Can you work these out from the model? Positions are in its coordinate system, mm. Face numbers are marked on the shaded views. A direction names the side the tool comes from. Coordinates: 2 decimals unless noted, no trailing zeros. Order: outer loops, then holes, each group sorted by start corner. A loop starts at its lowest first (then second) coordinate and runs counter-clockwise, first axis right, second up. Notation, with made-up numbers: (53, 89.5) -> (73, 89.5) arc R15 ccw to (73, 101.5) -> close; hole circle Ø4 at (-9.5, 71.5). An arc over 180 degrees is marked (long way). Answer in a Markdown table with one row per item. Add a question column.
1. Imagine slicing it at B-B on y = 6. Write out the boundary of the cut face in (x, z), plus the area to 3 significant figures.
2. Will these pins go through, and if not, where does the flat tip stop? pin 1 (4 mm diameter, centred on x = -31, z = -14.5, fed in from +Y); pin 2 (2 mm diameter, centred on x = -13, z = -16.5, fed in from +Y); pin 3 (1.1 mm diameter, centred on x = -31, z = 6, fed in from +Y); pin 4 (12 mm diameter, centred on x = 27, y = 19.5, fed in from +Z).
3. On a 3-axis mill with a long thin cutter (end or side, diameter ignored), from which of +Z, -Z, +X, -X, +Y, -Y can I reach the whole of each face in a straight line? I mean the marked faces 1, 2 and 3. Say none if no direction works.
4. Imagine slicing it at A-A on z = -1. Write out the boundary of the cut face in (x, y).
5. If I drill on line 1 along Z through (x, y) = (30.5, -4.25); line 2 along X through (y, z) = (-4, 5.4); line 3 along Z through (x, y) = (-29.5, -5), over which ranges is the centre line in solid material (lowest first)? Write a range as [from, to].
6. Imagine slicing it at D-D on x = 30.5. Write out the boundary of the cut face in (y, z).
7. We'd pull the mould along X, two halves only. Please class the marked faces 4, 5 and 6: pulls with the +X half, pulls with the -X half, needs draft (parallel to the pull), parting line crosses it, or undercut.
8. Imagine slicing it at C-C on x = 0. Write out the boundary of the cut face in (y, z), plus the area to 3 significant figures.
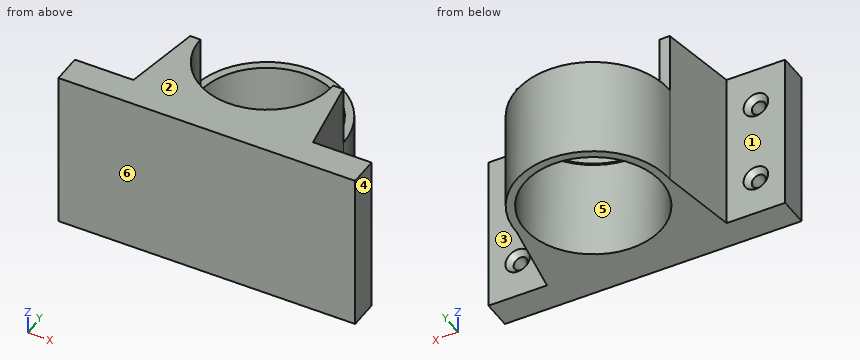
from build123d import *

# Parameters (mm, degrees)
SKETCH1_R                                       = 17.5
BOSS_EXTRUDE9_DEPTH                             = 25.5
BOSS_EXTRUDE10_DEPTH                            = 15.4
BOSS_EXTRUDE10_DEPTH_BACK                       = 25.5
CSK_FOR_M3_FLAT_HEAD_MACHINE_SCREW1_D           = 3.6
CSK_FOR_M3_FLAT_HEAD_MACHINE_SCREW1_CSINK_D     = 6.3
CSK_FOR_M3_FLAT_HEAD_MACHINE_SCREW1_CSINK_ANGLE = 90
CSK_FOR_M3_FLAT_HEAD_MACHINE_SCREW2_D           = 3.6
CSK_FOR_M3_FLAT_HEAD_MACHINE_SCREW2_CSINK_D     = 6.3
CSK_FOR_M3_FLAT_HEAD_MACHINE_SCREW2_CSINK_ANGLE = 90
BOSS_EXTRUDE11_DEPTH                            = 15.4
CUT_EXTRUDE3_REACH                              = 549.129
SKETCH17_R                                      = 1.8
SKETCH18_W                                      = 76
SKETCH18_H                                      = 40.9
BOSS_EXTRUDE12_DEPTH                            = 2.54


with BuildPart() as part:
    # Sketch1 → Boss-Extrude9 (new body)
    with BuildSketch(Plane.XY):
        with BuildLine():
            ThreePointArc((-19.6, 18.153395679), (0, 37.753395679), (19.6, 18.153395679))
            ThreePointArc((19.6, 18.153395679), (0, -1.446604321), (-19.6, 18.153395679))
        make_face()
        with Locations((0, 18.153395679)):
            Circle(SKETCH1_R, mode=Mode.SUBTRACT)
    extrude(amount=-BOSS_EXTRUDE9_DEPTH)

    # Sketch1<15> → Boss-Extrude10 (add, two sides: drawn at the far end of the back side and taken through both)
    with BuildSketch(Plane.XY.offset(-BOSS_EXTRUDE10_DEPTH_BACK)):
        with BuildLine():
            Line((-23, -1.846604321), (-38, -1.846604321))
            Line((-38, -1.846604321), (-38, -6.846604321))
            Line((-38, -6.846604321), (38, -6.846604321))
            Line((38, -6.846604321), (38, -1.846604321))
            Line((38, -1.846604321), (23, -1.846604321))
            Line((23, -1.846604321), (19.6, 18.153395679))
            ThreePointArc((19.6, 18.153395679), (0, -1.446604321), (-19.6, 18.153395679))
            Line((-19.6, 18.153395679), (-23, -1.846604321))
        make_face()
    extrude(amount=BOSS_EXTRUDE10_DEPTH + BOSS_EXTRUDE10_DEPTH_BACK)

    # CSK for M3 Flat Head Machine Screw1 (through all)
    with Locations(Plane(origin=(0, -1.846604321, 0), x_dir=(1, 0, 0), z_dir=(0, 1, 0))):
        with Locations((-30.5, 15.5), (-30.5, -5.4)):
            CounterSinkHole(CSK_FOR_M3_FLAT_HEAD_MACHINE_SCREW1_D / 2, CSK_FOR_M3_FLAT_HEAD_MACHINE_SCREW1_CSINK_D / 2, counter_sink_angle=CSK_FOR_M3_FLAT_HEAD_MACHINE_SCREW1_CSINK_ANGLE)

    # CSK for M3 Flat Head Machine Screw2 (through all)
    with Locations(Plane(origin=(0, -1.846604321, 0), x_dir=(1, 0, 0), z_dir=(0, 1, 0))):
        with Locations((30.5, -5.4), (30.5, 15.5)):
            CounterSinkHole(CSK_FOR_M3_FLAT_HEAD_MACHINE_SCREW2_D / 2, CSK_FOR_M3_FLAT_HEAD_MACHINE_SCREW2_CSINK_D / 2, counter_sink_angle=CSK_FOR_M3_FLAT_HEAD_MACHINE_SCREW2_CSINK_ANGLE)

    # Sketch1<19> → Boss-Extrude11 (add)
    with BuildSketch(Plane.XY):
        with BuildLine():
            ThreePointArc((-19.6, 18.153395679), (0, -1.446604321), (19.6, 18.153395679))
            Line((19.6, 18.153395679), (17, 18.153395679))
            ThreePointArc((17, 18.153395679), (0, 1.153395679), (-17, 18.153395679))
            Line((-17, 18.153395679), (-19.6, 18.153395679))
        make_face()
    extrude(amount=BOSS_EXTRUDE11_DEPTH)

    # Sketch17 → Cut-Extrude3 (cut, up to next)
    with BuildSketch(Plane(origin=(-499.24894984, 9.974554812, -84.308871479), x_dir=(0.050830850863694654, -0.0009181581696580717, 0.9987068546806156), z_dir=(0.0360908865319125, 0.9993480899541042, -0.0009181581696581681)), mode=Mode.PRIVATE) as cut_extrude3_sk1:
        with Locations((92.5, 462.5)):
            Circle(SKETCH17_R)
    cut_extrude3_tool1 = extrude(cut_extrude3_sk1.sketch, amount=-CUT_EXTRUDE3_REACH, mode=Mode.PRIVATE) & part.part
    # Sketch17 → Cut-Extrude3 (cut, up to next)
    with BuildSketch(Plane(origin=(-499.24894984, 9.974554812, -84.308871479), x_dir=(0.050830850863694654, -0.0009181581696580717, 0.9987068546806156), z_dir=(0.0360908865319125, 0.9993480899541042, -0.0009181581696581681)), mode=Mode.PRIVATE) as cut_extrude3_sk2:
        with Locations((113.4, 462.5)):
            Circle(SKETCH17_R)
    cut_extrude3_tool2 = extrude(cut_extrude3_sk2.sketch, amount=-CUT_EXTRUDE3_REACH, mode=Mode.PRIVATE) & part.part
    add(cut_extrude3_tool1.solids().sort_by_distance((-32.946684, -6.80241, -15.437756))[0], mode=Mode.SUBTRACT)
    add(cut_extrude3_tool2.solids().sort_by_distance((-31.884319, -6.821599, 5.435217))[0], mode=Mode.SUBTRACT)

    # Sketch18 → Boss-Extrude12 (add)
    with BuildSketch(Plane.XZ.offset(6.846604321)):
        with Locations((0, -5.05)):
            Rectangle(SKETCH18_W, SKETCH18_H)
    extrude(amount=BOSS_EXTRUDE12_DEPTH)


solid = part.part
Answers follow:
| question | item | result |
|---|---|---|
| 1 | outline | (-21.67, -25.5) -> (-12.59, -25.5) -> (-12.59, 0) -> (-11.89, 0) -> (-11.89, 15.4) -> (-21.67, 15.4) -> close; (11.89, 0) -> (12.59, 0) -> (12.59, -25.5) -> (21.67, -25.5) -> (21.67, 15.4) -> (11.89, 15.4) -> close |
| 1 | area | 764 mm² |
| 2 | pin 1 | stops at y = -1.88 |
| 2 | pin 2 | stops at y = 33.65 |
| 2 | pin 3 | stops at y = -6.85 |
| 2 | pin 4 | passes through |
| 3 | face 1 | +Z, -Z, -X, +Y |
| 3 | face 2 | +Z, +X, -X, +Y, -Y |
| 3 | face 3 | +Z, -Z, +X, +Y |
| 4 | outline | (-38, -9.39) -> (38, -9.39) -> (38, -1.85) -> (23, -1.85) -> (19.6, 18.15) arc R19.6 ccw to (-19.6, 18.15) -> (-23, -1.85) -> (-38, -1.85) -> close; hole circle Ø35 at (0, 18.15) |
| 5 | line 1 | z = [-25.5, -17.3], [-13.7, 3.6], [7.2, 15.4] |
| 5 | line 2 | x = [-38, -32.3], [-28.7, 28.7], [32.3, 38] |
| 5 | line 3 | z = [-25.5, -17], [-14, 3.9], [6.9, 15.4] |
| 6 | outline | (-9.39, -25.5) -> (-1.85, -25.5) -> (-1.85, -18.65) -> (-3.2, -17.3) -> (-6.85, -17.3) -> (-6.85, -13.7) -> (-3.2, -13.7) -> (-1.85, -12.35) -> (-1.85, 2.25) -> (-3.2, 3.6) -> (-6.85, 3.6) -> (-6.85, 7.2) -> (-3.2, 7.2) -> (-1.85, 8.55) -> (-1.85, 15.4) -> (-9.39, 15.4) -> close |
| 7 | face 4 | pulls with the +X half |
| 7 | face 5 | undercut |
| 7 | face 6 | needs draft |
| 8 | outline | (-9.39, -25.5) -> (0.65, -25.5) -> (0.65, 0) -> (1.15, 0) -> (1.15, 15.4) -> (-9.39, 15.4) -> close; (35.65, -25.5) -> (37.75, -25.5) -> (37.75, 0) -> (35.65, 0) -> close |
| 8 | area | 472 mm² |
